Build history of the part. All positions in model axes, mm. Face numbers are marked on the shaded views. A direction names the side the tool comes from. Give positions to 0.01 mm unless a question says otherwise; leave off trailing zeros. Order: outer loops, then holes, each group sorted by start corner. A loop starts at its lowest first (then second) coordinate and runs counter-clockwise, first axis right, second up. Notation, with made-up numbers: M 63,-18 L 86,-18 A24 ccw 86,2 Z; hole C 4.5,-19 d7. An arc over 180 degrees is marked long. One line per item, written item: value.
from build123d import *

# Parameters (mm, degrees)
SKETCH_R        = 3
PAD_DEPTH       = 5
SKETCH001_W     = 15.685142
SKETCH001_H     = 2
POCKET_DEPTH    = 4
SKETCH002_R     = 1.75
PAD001_DEPTH    = 10
SKETCH003_W     = 8.687401
SKETCH003_H     = 3.263626
POCKET001_DEPTH = 4
CHAMFER_SIZE    = 0.5


with BuildPart() as part:
    # Sketch → Pad (new body)
    with BuildSketch(Plane(origin=(0, 0, 0), x_dir=(0, 1, 0), z_dir=(0, 0, 1))):
        Circle(SKETCH_R)
    extrude(amount=PAD_DEPTH)

    # Sketch001 → Pocket (cut)
    with BuildSketch(Plane.XY.offset(5)):
        Rectangle(SKETCH001_W, SKETCH001_H)
    extrude(amount=-POCKET_DEPTH, mode=Mode.SUBTRACT)

    # Sketch002 → Pad001 (join)
    with BuildSketch(Plane(origin=(0, 0, 0), x_dir=(0, 1, 0), z_dir=(0, 0, 1))):
        Circle(SKETCH002_R)
    extrude(amount=PAD001_DEPTH)

    # Sketch003 → Pocket001 (cut)
    with BuildSketch(Plane.XY.offset(10)):
        with Locations((-0.081454, 2.331813)):
            Rectangle(SKETCH003_W, SKETCH003_H)
    extrude(amount=-POCKET001_DEPTH, mode=Mode.SUBTRACT)

    # Chamfer
    chamfer_edges = [part.edges().sort_by_distance(p)[0] for p in [
        (0, -1.75, 10),
        (0, -3, 5),
        (-1.732051, 2.44949, 5),
        (1.732051, 2.44949, 5),
    ]]
    chamfer(chamfer_edges, length=CHAMFER_SIZE)


solid = part.part
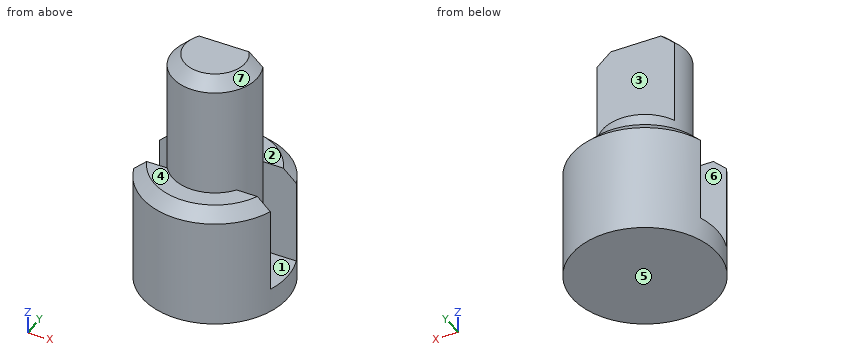
1) Drill centre lines: probe 1 along Z at (x, y) = (2.75, 0.4); probe 2 along X at (y, z) = (0.05, 3.5); probe 3 along Z at (x, y) = (0.55, 2.1). Where is each one in solid material? Low to high. Write a range as from..to.
Check values:
probe 1: 0..1
probe 2: -1.75..1.75
probe 3: 0..5
2) Saw through at A-A, the plane z = 3. Write the cut outline in (x, y).
Check values:
outline: M -2.83,-1 A3 ccw 2.83,-1 L 1.44,-1 A1.75 ccw 1.44,1 L 2.83,1 A3 ccw -2.83,1 L -1.44,1 A1.75 ccw -1.44,-1 Z
3) Saw through at B-B, the plane x = 0. Write the cut outline in (y, z).
Check values:
outline: M -3,0 L 3,0 L 3,4.5 L 2.5,5 L 1.75,5 L 1.75,6 L 0.7,6 L 0.7,10 L -1.25,10 L -1.75,9.5 L -1.75,5 L -2.5,5 L -3,4.5 Z
4) Saw through at C-C, the plane y = 0. Write the cut outline in (x, z).
Check values:
outline: M -3,0 L 3,0 L 3,1 L 1.75,1 L 1.75,9.5 L 1.25,10 L -1.25,10 L -1.75,9.5 L -1.75,1 L -3,1 Z
5) Mould opens along Y. For the marked faces 5, 6 and 7 say: released by +Y, released by -Y, zero draft, split by the parting line, or undercut.
Check values:
face 5: zero draft
face 6: undercut
face 7: split by the parting line
6) Tool access for the marked faces 1, 2, 3 and 4: list every direction of +Z, -Z, +X, -X, +Y, -Y with a clear straight run to the whole face (end or side of a thin tool).
Check values:
face 1: +Z, +X
face 2: +Z, +Y
face 3: +Z, +X, -X, +Y
face 4: +Z, -Y
7) Saw through at D-D, the plane z = 7.25. Write the cut outline in (x, y), then the cut area to 3 significant figures.
Check values:
outline: M -1.6,0.7 A1.75 ccw long 1.6,0.7 Z
area: 7.19 mm^2
8) Pin check, flat tips, straight feed: pin 1 (1 mm diameter, centred on x = -2, y = 0.5, fed in from +Z); pin 2 (1.2 mm diameter, centred on x = 0, y = 1.5, fed in from +Z); pin 3 (0.8 mm diameter, centred on x = -2, y = -0.5, fed in from +Z). Stop position of each tip, or through.
Check values:
pin 1: z = 9.69
pin 2: z = 6
pin 3: z = 9.59
